Build history of the part. All positions in model axes, mm. Give positions to 0.01 mm unless a question says otherwise; leave off trailing zeros. Loops run counter-clockwise (first coordinate to the right, second up) from the corner with the lowest first, then second, coordinate; pieces in that order, holes last. Notation, with made-up numbers: (42.5, 20) -> (81.5, 20) arc R11 cw to (81.5, 36) -> close; hole circle Ø8 at (-32, 45.25). An arc over 180 degrees is marked (long way). Answer as a JSON object with one key per item and string values. Group by question number.
Q1. Band-saw the part on A-A, the plane x = -5.5. Write the cut outline in (y, z).
Q2. Band-saw the part on B-B, the plane z = 38.1. Write the cut outline in (x, y) (1 decimal).
Q3. Band-saw the part on C-C, the plane y = 0. Write the cut outline in (x, z).
Q4. Band-saw the part on D-D, the plane z = 109. Write the cut outline in (x, y).
Q5. Wall check: probe 1 along Y at (x, z) = (-4, 15); probe 2 along X at (y, z) = (12.2, 190.5); probe 3 along X at (y, z) = (-12.2, 38.1) (3 decimals). Give the ranges that are in metal, low to high. Write a range as from..to.
Q6. Drop a flat-ended pin along its axis: pin 1 (3.5 mm diameter, centred on x = 0, z = 241.3, fed in from -Y). Give the stop position or say it passes through.
from build123d import *

# Parameters (mm, degrees)
SKETCH1_W           = 25.4
SKETCH1_H           = 25.4
SKETCH1_W_2         = 22.225
SKETCH1_H_2         = 22.225
BOSS_EXTRUDE1_DEPTH = 279.4
SKETCH2_R           = 1.984375
CUT_EXTRUDE1_DEPTH  = 26.4
SKETCH3_R           = 3.175
CUT_EXTRUDE2_DEPTH  = 26.4
SKETCH4_R           = 6.35
CUT_EXTRUDE3_DEPTH  = 26.4


with BuildPart() as part:
    # Sketch1 → Boss-Extrude1 (new body)
    with BuildSketch(Plane.XY):
        Rectangle(SKETCH1_W, SKETCH1_H)
        Rectangle(SKETCH1_W_2, SKETCH1_H_2, mode=Mode.SUBTRACT)
    extrude(amount=BOSS_EXTRUDE1_DEPTH)

    # Sketch2 → Cut-Extrude1 (cut, through all)
    with BuildSketch(Plane(origin=(0, 12.7, 0), x_dir=(1, 0, 0), z_dir=(0, 1, 0))):
        with Locations((0, -266.7)):
            Circle(SKETCH2_R)
        with Locations((0, -241.3)):
            Circle(SKETCH2_R)
        with Locations((0, -215.9)):
            Circle(SKETCH2_R)
        with Locations((0, -190.5)):
            Circle(SKETCH2_R)
        with Locations((0, -165.1)):
            Circle(SKETCH2_R)
        with Locations((0, -139.7)):
            Circle(SKETCH2_R)
        with Locations((0, -114.3)):
            Circle(SKETCH2_R)
        with Locations((0, -88.9)):
            Circle(SKETCH2_R)
        with Locations((0, -63.5)):
            Circle(SKETCH2_R)
        with Locations((0, -38.1)):
            Circle(SKETCH2_R)
        with Locations((0, -12.7)):
            Circle(SKETCH2_R)
        with Locations((0, 12.7)):
            Circle(SKETCH2_R)
    extrude(amount=-CUT_EXTRUDE1_DEPTH, mode=Mode.SUBTRACT)

    # Sketch3 → Cut-Extrude2 (cut, through all)
    with BuildSketch(Plane(origin=(0, 12.7, 0), x_dir=(1, 0, 0), z_dir=(0, 1, 0))):
        with Locations((0, -38.1)):
            Circle(SKETCH3_R)
    extrude(amount=-CUT_EXTRUDE2_DEPTH, mode=Mode.SUBTRACT)

    # Sketch4 → Cut-Extrude3 (cut, through all)
    with BuildSketch(Plane(origin=(12.7, 0, 0), x_dir=(0, 0, -1), z_dir=(1, 0, 0))):
        with Locations((-12.7, 0)):
            Circle(SKETCH4_R)
    extrude(amount=-CUT_EXTRUDE3_DEPTH, mode=Mode.SUBTRACT)


solid = part.part
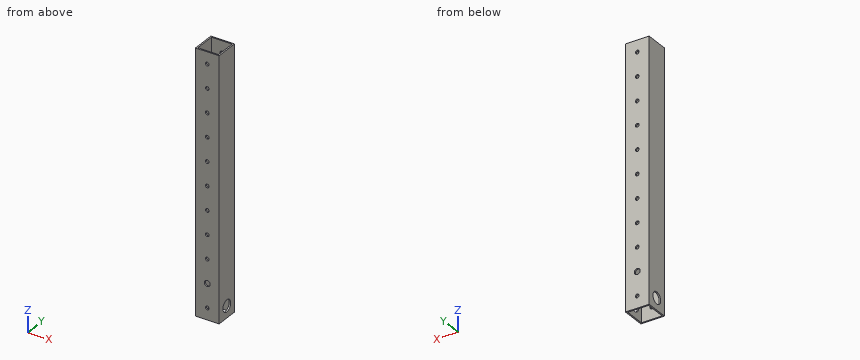
Worked answers:
{
 "1": {"outline": "(-12.7, 0) -> (-11.11, 0) -> (-11.11, 279.4) -> (-12.7, 279.4) -> close; (11.11, 0) -> (12.7, 0) -> (12.7, 279.4) -> (11.11, 279.4) -> close"},
 "2": {"outline": "(-12.7, -12.7) -> (-3.2, -12.7) -> (-3.2, -11.1) -> (-11.1, -11.1) -> (-11.1, 11.1) -> (-3.2, 11.1) -> (-3.2, 12.7) -> (-12.7, 12.7) -> close; (3.2, -12.7) -> (12.7, -12.7) -> (12.7, 12.7) -> (3.2, 12.7) -> (3.2, 11.1) -> (11.1, 11.1) -> (11.1, -11.1) -> (3.2, -11.1) -> close"},
 "3": {"outline": "(-12.7, 0) -> (-11.11, 0) -> (-11.11, 6.35) -> (-12.7, 6.35) -> close; (-12.7, 19.05) -> (-11.11, 19.05) -> (-11.11, 279.4) -> (-12.7, 279.4) -> close; (11.11, 0) -> (12.7, 0) -> (12.7, 6.35) -> (11.11, 6.35) -> close; (11.11, 19.05) -> (12.7, 19.05) -> (12.7, 279.4) -> (11.11, 279.4) -> close"},
 "4": {"outline": "(-12.7, -12.7) -> (12.7, -12.7) -> (12.7, 12.7) -> (-12.7, 12.7) -> close; hole (-11.11, -11.11) -> (11.11, -11.11) -> (11.11, 11.11) -> (-11.11, 11.11) -> close"},
 "5": {"probe 1": "-12.7..-11.11, 11.11..12.7", "probe 2": "-12.7..-1.98, 1.98..12.7", "probe 3": "-12.7..-3.175, 3.175..12.7"},
 "6": {"pin 1": "through"}
}
